Geometry: final body of the model. Coordinates: model frame, mm. A direction names the side the tool comes from. Round coordinates to 2 decimals unless told otherwise and drop trailing zeros. Loops run counter-clockwise (first coordinate to the right, second up) from the corner with the lowest first, then second, coordinate; pieces in that order, holes last. Notation, with made-up numbers: M -39.5,28.25 L -4.5,28.25 A15 ccw -4.5,56.25 Z; hole C -20.5,68.5 d1. An arc over 180 degrees is marked long. Answer as a JSON object with one key per item and string values.
```python
from build123d import *

# Parameters (mm, degrees)
F0_W     = 101.6
F0_H     = 76.2
F1_DEPTH = 12.7
F4_D     = 12.7
F5_W     = 11.43
F5_H     = 31.75
F7_W     = 19.05
F7_H     = 12.7
F9_W     = 19.05
F9_H     = 12.7
F11_R    = 2.54
F12_SIZE = 2.54


with BuildPart() as f1:
    # F0 (on Top) → F1 (new body)
    with BuildSketch(Plane.XY):
        Rectangle(F0_W, F0_H)
    extrude(amount=F1_DEPTH)

    # F4 (through all)
    with Locations(Plane.XY.offset(12.7)):
        with Locations((-41.501624, 27.920099), (41.256946, 27.920099), (41.256946, -27.920099), (-41.501624, -27.920099)):
            Hole(F4_D / 2)

    # F5 (on Front) → F6 (revolve)
    with BuildSketch(Plane.XZ):
        with Locations((5.715, 28.575)):
            Rectangle(F5_W, F5_H)
    revolve(axis=Axis((0, 0, 28.575), (0, 0, 1)))

    # F7 (on Front) → F8 (revolve)
    with BuildSketch(Plane.XZ):
        with Locations((9.525, 19.05)):
            Rectangle(F7_W, F7_H)
    revolve(axis=Axis((0, 0, 19.05), (0, 0, 1)))

    # F9 (on Front) → F10 (revolve)
    with BuildSketch(Plane.XZ):
        with Locations((9.525, 43.846787)):
            Rectangle(F9_W, F9_H)
    revolve(axis=Axis((0, 0, 43.846787), (0, 0, 1)))

    # F11
    f11_edges = [f1.edges().sort_by_distance(p)[0] for p in [
        (-19.05, 0, 50.196787),
        (-19.05, 0, 12.7),
    ]]
    fillet(f11_edges, radius=F11_R)

    # F12
    f12_edges = [f1.edges().sort_by_distance(p)[0] for p in [
        (0, 38.1, 12.7),
        (50.8, 0, 12.7),
        (0, -38.1, 12.7),
        (-50.8, 0, 12.7),
    ]]
    chamfer(f12_edges, length=F12_SIZE)


solid = f1.part
```
1) Cut plane A-A on y = 0. Return the cut outline in (x, z).
Geometry results:
{"outline": "M -50.8,0 L 50.8,0 L 50.8,10.16 L 48.26,12.7 L 21.59,12.7 A2.54 cw 19.05,15.24 L 19.05,25.4 L 11.43,25.4 L 11.43,37.5 L 19.05,37.5 L 19.05,47.66 A2.54 ccw 16.51,50.2 L -16.51,50.2 A2.54 ccw -19.05,47.66 L -19.05,37.5 L -11.43,37.5 L -11.43,25.4 L -19.05,25.4 L -19.05,15.24 A2.54 cw -21.59,12.7 L -48.26,12.7 L -50.8,10.16 Z"}
2) Line query: probe 1 along Y at (x, z) = (43, 2); probe 2 along Z at (x, y) = (13.5, -4.5); probe 3 along X at (y, z) = (-24.5, 8). Output: solid intervals per line, ascending.
Geometry results:
{"probe 1": "-38.1 to -34.03, -21.81 to 21.81, 34.03 to 38.1", "probe 2": "0 to 25.4, 37.5 to 50.2", "probe 3": "-50.8 to -46.85, -36.15 to 35.91, 46.61 to 50.8"}
3) First-contact query: pin 1 (3 mm diameter, centred on y = -8, z = 42, fed in from -X); pin 2 (1.5 mm diameter, centred on x = -38.5, y = 14, fed in from +Z); pin 3 (2 mm diameter, centred on y = 12, z = 14.5, fed in from -X). Flat tips, straight axial feed; report the tip coordinate or a pass-through.
Geometry results:
{"pin 1": "x = -17.91", "pin 2": "z = 12.7", "pin 3": "x = -15.91"}
4) Set-up query: faces 1 (the face through (-8.2, -8.2, 37.497)), 2 (the face through (-15.12, -11.59, 42.65)), 3 (the face through (-1, 1, 0)). Return all of +Z, -Z, +X, -X, +Y, -Y with unobstructed straight access to the full face (end or side cutting, diameter ignored); none if empty.
Geometry results:
{"face 1": "none", "face 2": "+Z", "face 3": "-Z, +X, -X, +Y, -Y"}
5) Cut plane B-B on x = 0. Return the cut outline in (y, z), and give its area (3 significant figures).
Geometry results:
{"outline": "M -38.1,0 L 38.1,0 L 38.1,10.16 L 35.56,12.7 L 21.59,12.7 A2.54 cw 19.05,15.24 L 19.05,25.4 L 11.43,25.4 L 11.43,37.5 L 19.05,37.5 L 19.05,47.66 A2.54 ccw 16.51,50.2 L -16.51,50.2 A2.54 ccw -19.05,47.66 L -19.05,37.5 L -11.43,37.5 L -11.43,25.4 L -19.05,25.4 L -19.05,15.24 A2.54 cw -21.59,12.7 L -35.56,12.7 L -38.1,10.16 Z", "area": "2,210 mm2"}
6) Cut plane C-C on z = 6. Return the cut outline in (x, y).
Geometry results:
{"outline": "M -50.8,-38.1 L 50.8,-38.1 L 50.8,38.1 L -50.8,38.1 Z; hole C -41.5,-27.92 d12.7; hole C -41.5,27.92 d12.7; hole C 41.26,-27.92 d12.7; hole C 41.26,27.92 d12.7"}
7) Pull-direction query (Z, two-part tool) for faces 4 (the face through (-36.46, -31.78, 6.26)), 5 (the face through (49.55, -0.53, 11.41)), 6 (the face through (-8.2, -8.2, 25.4)), 7 (the face through (10.902, 3.433, 31.533)); classes: +Z half, -Z half, draft (parallel to the pull), parting line (faces both ways), or undercut.
Geometry results:
{"face 4": "draft", "face 5": "+Z half", "face 6": "undercut", "face 7": "undercut"}
8) Cut plane D-D on z = 35.5. Return the cut outline in (x, y).
Geometry results:
{"outline": "C 0,0 d22.86"}
